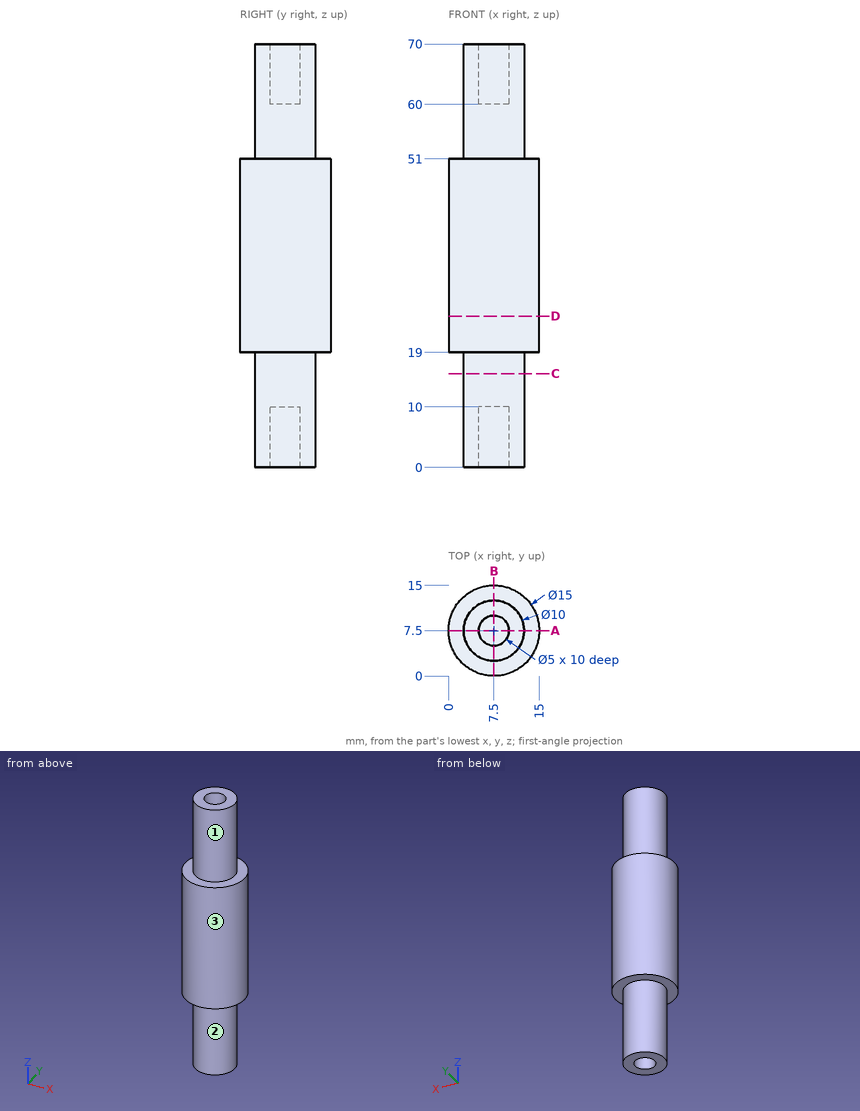
Geometry check sheet. Reference: drawing and pictorial views, mm from the part's lowest x, y, z. A direction names the side the tool comes from. Round coordinates to 2 decimals unless told otherwise and drop trailing zeros. Loops run counter-clockwise (first coordinate to the right, second up) from the corner with the lowest first, then second, coordinate; pieces in that order, holes last. Notation, with made-up numbers: M 34.25,37 L 40.25,37 A12 cw 40.25,57 Z; hole C 68.5,-30 d10. An arc over 180 degrees is marked long. Return JSON: item names as keys, results as strings. Group by question number.
(1) Section check A-A, the plane y = 7.5. Enter the section's corners in (x, z), and give its area (3 significant figures).
(2) Set-up check for the marked faces 1, 2 and 3: record each of +Z, -Z, +X, -X, +Y, -Y from which the full face is reachable in a straight line by a thin tool's end or side.
(3) Section check C-C, the plane z = 15.5. Enter the section's corners in (x, y).
(4) Section check D-D, the plane z = 25. Enter the section's corners in (x, y), and give its area (3 significant figures).
(5) Scan lines: line 1 along Y through (x, z) = (7.5, 67.75); line 2 along Z through (x, y) = (13.5, 3.25); line 3 along X through (y, z) = (5.5, 61.5). Record each from-to range of solid material in increasing order. Write a range as [from, to].
(6) Go/stop test with flat-tipped pins: pin 1 (6 mm diameter, centred on x = 4.5, z = 9.5, fed in from -Y); pin 2 (4 mm diameter, centred on x = 7.5, y = 7.5, fed in from +Z); pin 3 (5 mm diameter, centred on y = 2.5, z = 45.5, fed in from -X). Record where each tip stops, or that it passes through.
Data:
{
 "1": {"outline": "M 0,19 L 2.5,19 L 2.5,0 L 5,0 L 5,10 L 10,10 L 10,0 L 12.5,0 L 12.5,19 L 15,19 L 15,51 L 12.5,51 L 12.5,70 L 10,70 L 10,60 L 5,60 L 5,70 L 2.5,70 L 2.5,51 L 0,51 Z", "area": "760 mm²"},
 "2": {"face 1": "+Z", "face 2": "-Z", "face 3": "+Z, -Z"},
 "3": {"outline": "C 7.5,7.5 d10"},
 "4": {"outline": "C 7.5,7.5 d15", "area": "177 mm²"},
 "5": {"line 1": "[2.5, 5], [10, 12.5]", "line 2": "[19, 51]", "line 3": "[2.92, 6], [9, 12.08]"},
 "6": {"pin 1": "y = 2.5", "pin 2": "z = 60", "pin 3": "x = 0.43"}
}
